Check sheet for the drawn part. Datum: minimum x, y, z corner. Units: mm. Coordinates: 2 decimals unless noted, no trailing zeros. Order: outer loops, then holes, each group sorted by start corner. A loop starts at its lowest first (then second) coordinate and runs counter-clockwise, first axis right, second up.
Q1. Cross-section at A-A, the plane x = 63.75. Record the boundary of the cut face in (y, z).
Q2. Cross-section at C-C, the plane y = 12.25. Count the separate pieces of the cut face and the enclosed holes in it, and give its area (4 significant figures).
Q3. Cross-section at B-B, the plane z = 1.05. Record the boundary of the cut face in (x, y), and give its area (3 significant figures).
Q4. Cross-section at D-D, the plane x = 19.75. Record the boundary of the cut face in (y, z), and give its area (4 significant figures).
Q5. Depth check by flat-ended pin: P1, Ø6, axis at x = 18, y = 13.5, coming from the -Z side. Enter the tip coordinate at first touch or a pass-through.
Q6. Thickness scan on line 1 (X direction, y = 11.5, z = 0.85); line 2 (X direction, y = 17.25, z = 1.2); line 3 (X direction, y = 14, z = 1.3). Record the ranges inside material, lowest first.
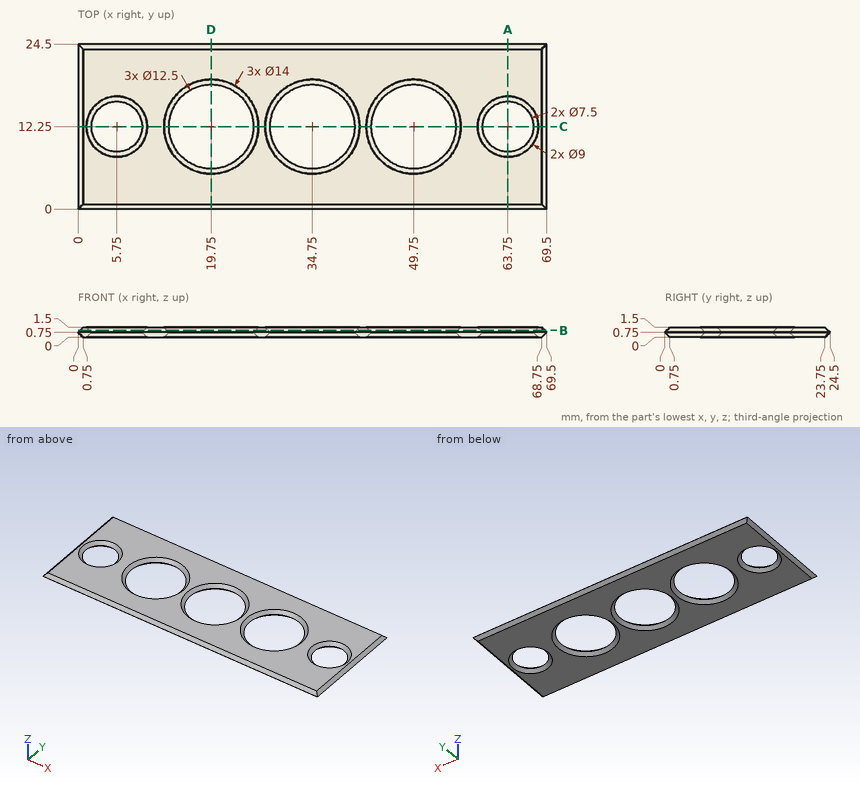
Check values:
1. outline: (0, 0.75) - (0.75, 0) - (7.75, 0) - (8.5, 0.75) - (7.75, 1.5) - (0.75, 1.5) - close; (16, 0.75) - (16.75, 0) - (23.75, 0) - (24.5, 0.75) - (23.75, 1.5) - (16.75, 1.5) - close
2. separate pieces: 6
2. enclosed holes: 0
2. area: 18.75 mm2
3. outline: (0.3, 0.3) - (69.2, 0.3) - (69.2, 24.2) - (0.3, 24.2) - close; hole circle Ø8.1 at (5.75, 12.25); hole circle Ø13.1 at (19.75, 12.25); hole circle Ø13.1 at (34.75, 12.25); hole circle Ø13.1 at (49.75, 12.25); hole circle Ø8.1 at (63.75, 12.25)
3. area: 1,140 mm2
4. outline: (0, 0.75) - (0.75, 0) - (5.25, 0) - (6, 0.75) - (5.25, 1.5) - (0.75, 1.5) - close; (18.5, 0.75) - (19.25, 0) - (23.75, 0) - (24.5, 0.75) - (23.75, 1.5) - (19.25, 1.5) - close
4. area: 15.75 mm2
5. P1: passes through
6. line 1: x = 0.1 to 1.97, 9.53 to 13.44, 26.06 to 28.44, 41.06 to 43.44, 56.06 to 59.97, 67.53 to 69.4
6. line 2: x = 0.45 to 15.29, 24.21 to 30.29, 39.21 to 45.29, 54.21 to 69.05
6. line 3: x = 0.55 to 1.82, 9.68 to 13.18, 26.32 to 28.18, 41.32 to 43.18, 56.32 to 59.82, 67.68 to 68.95
